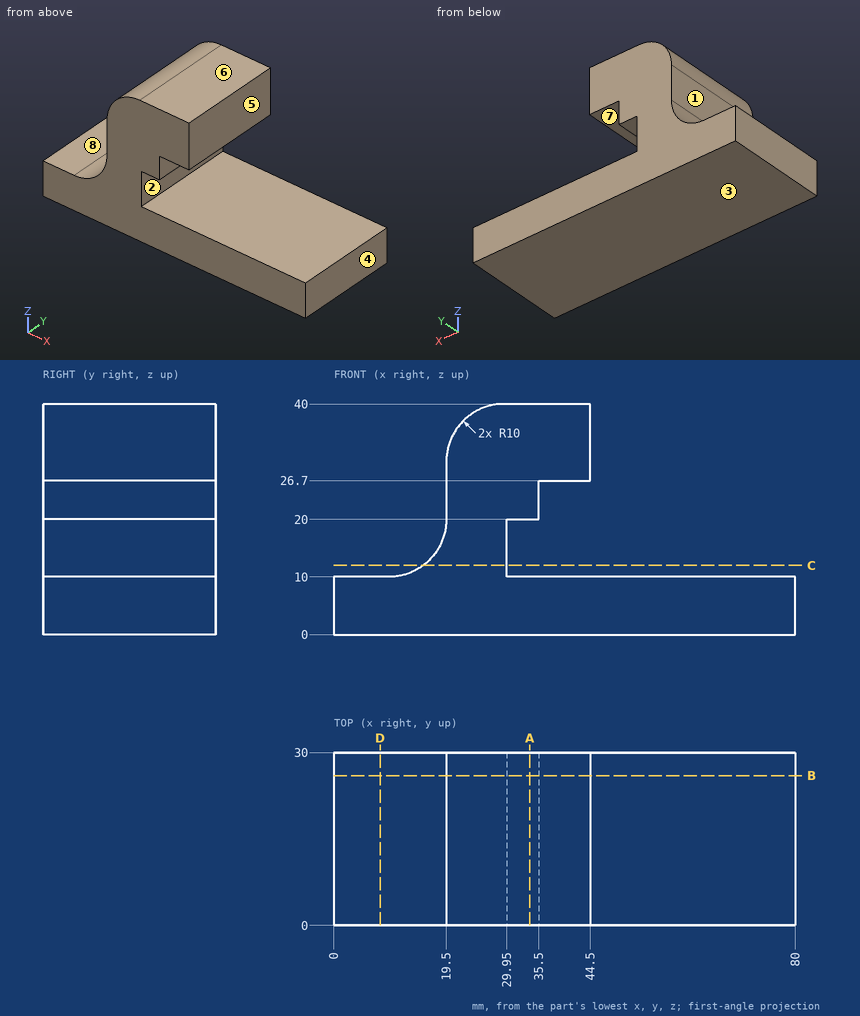
Could you check a few things on this drawing? It's one solid part, dimensions in mm from its lowest x, y, z. A direction names the side the tool comes from. Coordinates: 2 decimals unless noted, no trailing zeros. Order: outer loops, then holes, each group sorted by start corner. A loop starts at its lowest first (then second) coordinate and runs counter-clockwise, first axis right, second up. Notation, with made-up numbers: M -9.5,65.25 L 25.5,65.25 A14 cw 25.5,78.25 Z; hole C 84.25,-26 d6. An arc over 180 degrees is marked long. Use one line per item in the form item = value. Start each with the question number.
1. We'd pull the mould along Z, two halves only. Please class the marked faces 1, 2 and 3: +Z half, -Z half, draft (parallel to the pull), parting line (faces both ways), or undercut.
2. Please list where these lines run through material, in increasing order: line 1 (Z direction, x = 39.5, y = 17); line 2 (Z direction, x = 75, y = 26.25); line 3 (X direction, y = 9.5, z = 22.5).
3. Suppose I cut it at D-D on x = 8. Write out the boundary of the cut face in (y, z), then the cut area to 3 significant figures.
4. Suppose I cut it at B-B on y = 26. Write out the boundary of the cut face in (x, z).
5. For pin 1 (3 mm diameter, centred on y = 18.5, z = 13.5, fed in from +X); pin 2 (3 mm diameter, centred on y = 22.5, z = 27.5, fed in from -X); pin 3 (6.5 mm diameter, centred on y = 18, z = 33, fed in from +X); pin 4 (1 mm diameter, centred on y = 6.5, z = 7.5, fed in from -X), each with a flat end and sliding along its axis, tell me the tip position at first contact or that it passes through.
6. Suppose I cut it at A-A on x = 34. Write out the boundary of the cut face in (y, z).
7. On a 3-axis mill with a long thin cutter (end or side, diameter ignored), from which of +Z, -Z, +X, -X, +Y, -Y can I reach the whole of each face in a straight line? I mean the marked faces 4, 5, 6, 7 and 8. Say none if no direction works.
8. Suppose I cut it at C-C on z = 12. Write out the boundary of the cut face in (x, y), then the cut area to 4 significant figures.
Geometry says:
q1.face_1 = draft
q1.face_2 = undercut
q1.face_3 = -Z half
q2.line_1 = 0 to 10, 26.7 to 40
q2.line_2 = 0 to 10
q2.line_3 = 19.5 to 35.5
q3.outline = M 0,0 L 30,0 L 30,10 L 0,10 Z
q3.area = 300 mm^2
q4.outline = M 0,0 L 80,0 L 80,10 L 29.95,10 L 29.95,20 L 35.5,20 L 35.5,26.7 L 44.5,26.7 L 44.5,40 L 29.5,40 A10 ccw 19.5,30 L 19.5,20 A10 cw 9.5,10 L 0,10 Z
q5.pin_1 = 29.95
q5.pin_2 = 19.5
q5.pin_3 = 44.5
q5.pin_4 = 0
q6.outline = M 0,0 L 30,0 L 30,10 L 0,10 Z; M 0,20 L 30,20 L 30,40 L 0,40 Z
q7.face_4 = +Z, -Z, +X, +Y, -Y
q7.face_5 = +Z, +X, +Y, -Y
q7.face_6 = +Z, +X, -X, +Y, -Y
q7.face_7 = +X, +Y, -Y
q7.face_8 = +Z, -X, +Y, -Y
q8.outline = M 15.5,0 L 29.95,0 L 29.95,30 L 15.5,30 Z
q8.area = 433.5 mm^2
